Geometry: final body of the model. Coordinates: model frame, mm. A direction names the side the tool comes from. Give positions to 0.01 mm unless a question says otherwise; leave off trailing zeros. Loops run counter-clockwise (first coordinate to the right, second up) from the corner with the lowest first, then second, coordinate; pieces in that order, holes last. Notation, with made-up numbers: (74, -28.5) -> (115, -28.5) arc R24 cw to (115, -17.5) -> close; hole circle Ø4 at (85.25, 3.25). An arc over 180 degrees is marked (long way). Answer in a Markdown table with one row per item. Add a question column.
1) Draft query along X for faces 5 (the flat face through (0, -2, 16.095)), 6 (the cylindrical face through (12.933, -2.379, -0.262)), 7 (the flat face through (-6.35, -2, 14)), 8 (the cylindrical face through (-2.539, -2.379, -1.947)). Return one class per face: +X half, -X half, draft (parallel to the pull), parting line (faces both ways), or undercut.
2) Line query: line 1 (X direction, y = -2.2, z = -1); line 2 (Z direction, x = 0, y = -1.4); line 3 (Z direction, x = -20, y = -4.05). Output: solid intervals per line, ascending. Write a range as from..to.
3) Section query C-C (x = 0). Return the cut outline in (y, z).
4) Section query B-B (y = -0.75). Give the number of separate pieces and of enclosed holes in the cut face, plus the area to 3 significant figures.
5) Access query for faces 1 (the flat face through (-21, -2, -11.337)), 2 (the flat face through (6.35, -2.38, -13.78)), 3 (the flat face through (-21, -2, 11.269)), 4 (the flat face through (6.35, -2, 14)). Directions: +Z, -Z, +X, -X, +Y, -Y. A direction counts if a zero-diameter tool reaches every point of the face in a straight line with its end or side. Return the directions, or none.
6) Section query D-D (x = -22). Return the cut outline in (y, z), plus the area to 3 significant figures.
7) First-contact query: P1, Ø12, axis at x = 7.5, z = -10, coming from the +Y side; P2, Ø2.5, axis at x = -12.319, z = 0, coming from the -Y side (1 decimal); P3, Ø1.4, axis at x = -19, y = -2.5, coming from the -Z side; P4, Ø1.4, axis at y = -3, z = 14, coming from the -X side. Flat tips, straight axial feed; report the tip coordinate or a pass-through.
8) Section query A-A (z = 0). Return the cut outline in (x, y).
```python
from build123d import *

# Parameters (mm, degrees)
F0_R     = 1.905
F0_R_2   = 3.2
F1_DEPTH = 4.826


# Not quite as in the source:
# - a feature names something its author has since deleted; it is built from what else it names


with BuildPart() as f1:
    # F0 (on Front) → F1 (new body)
    with BuildSketch(Plane.XZ):
        with BuildLine():
            Line((-6.2288098753, -16.020498732), (6.4704601492, -16.156663498))
            Line((6.4704601492, -16.156663498), (6.2288098753, -11.3367173214))
            ThreePointArc((6.2288098753, -11.3367173214), (12.9350076718, -0.0693442092), (6.35, 11.2692826786))
            Line((6.35, 11.2692826786), (6.35, 16.0952826786))
            Line((6.35, 16.0952826786), (-6.35, 16.0952826786))
            Line((-6.35, 16.0952826786), (-6.35, 11.2692826786))
            Line((-6.35, 11.2692826786), (-35.56, 11.2692826786))
            Line((-35.56, 11.2692826786), (-35.56, -11.3367173214))
            Line((-35.56, -11.3367173214), (-6.4636334645, -11.3367173214))
            Line((-6.4636334645, -11.3367173214), (-6.2288098753, -16.020498732))
        make_face()
        with Locations((-12.319, 0)):
            Circle(F0_R, mode=Mode.SUBTRACT)
        Circle(F0_R_2, mode=Mode.SUBTRACT)
    extrude(amount=F1_DEPTH)


solid = f1.part
```
Evaluation:
| question | item | result |
|---|---|---|
| 1 | face 5 | draft |
| 1 | face 6 | +X half |
| 1 | face 7 | -X half |
| 1 | face 8 | undercut |
| 2 | line 1 | -35.56..-13.94, -10.7..-3.04, 3.04..12.9 |
| 2 | line 2 | -16.09..-3.2, 3.2..16.1 |
| 2 | line 3 | -11.34..11.27 |
| 3 | outline | (-4.83, -16.09) -> (0, -16.09) -> (0, -3.2) -> (-4.83, -3.2) -> close; (-4.83, 3.2) -> (0, 3.2) -> (0, 16.1) -> (-4.83, 16.1) -> close |
| 4 | separate pieces | 1 |
| 4 | enclosed holes | 2 |
| 4 | area | 1,130 mm² |
| 5 | face 1 | -Z, -X, +Y, -Y |
| 5 | face 2 | +X, +Y, -Y |
| 5 | face 3 | +Z, -X, +Y, -Y |
| 5 | face 4 | +Z, +X, +Y, -Y |
| 6 | outline | (-4.83, -11.34) -> (0, -11.34) -> (0, 11.27) -> (-4.83, 11.27) -> close |
| 6 | area | 109 mm² |
| 7 | P1 | y = 0 |
| 7 | P2 | through |
| 7 | P3 | z = -11.34 |
| 7 | P4 | x = -6.35 |
| 8 | outline | (-35.56, -4.83) -> (-14.22, -4.83) -> (-14.22, 0) -> (-35.56, 0) -> close; (-10.41, -4.83) -> (-3.2, -4.83) -> (-3.2, 0) -> (-10.41, 0) -> close; (3.2, -4.83) -> (12.94, -4.83) -> (12.94, 0) -> (3.2, 0) -> close |
